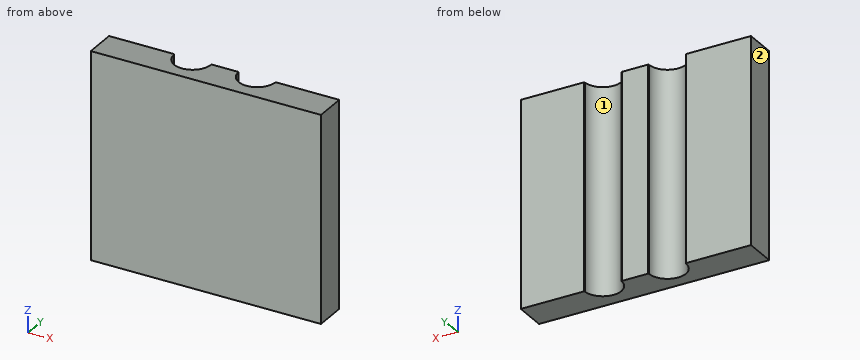
```python
from build123d import *

# Parameters (mm, degrees)
SKETCH1_W           = 38
SKETCH1_H           = 34
BOSS_EXTRUDE1_DEPTH = 2
BOSS_EXTRUDE2_DEPTH = 34
CHAMFER1_SIZE       = 0.1
CHAMFER1_SIZE_2     = 0.100939666
CHAMFER1_SIZE_3     = 0.096996068


with BuildPart() as part:
    # Sketch1 → Boss-Extrude1 (new body)
    with BuildSketch(Plane(origin=(0, 0, 0), x_dir=(1, 0, 0), z_dir=(0, 1, 0))):
        Rectangle(SKETCH1_W, SKETCH1_H)
    extrude(amount=BOSS_EXTRUDE1_DEPTH)

    # Sketch2 → Boss-Extrude2 (add, through all)
    with BuildSketch(Plane.XY.offset(17)):
        with BuildLine():
            Line((-2.101169585, 5.192456713), (2.394541693, 5.192456713))
            ThreePointArc((2.394541693, 5.192456713), (5.447861319, 2.177768465), (8.494206352, 5.199504374))
            Line((8.494206352, 5.199504374), (19, 5.199504374))
            Line((19, 5.199504374), (19, 1.662378765))
            Line((19, 1.662378765), (-19, 1.662378765))
            Line((-19, 1.662378765), (-19, 5.198537403))
            Line((-19, 5.198537403), (-8.197951747, 5.198537403))
            ThreePointArc((-8.197951747, 5.198537403), (-5.152701361, 2.046490686), (-2.101169585, 5.192456713))
        make_face()
    extrude(amount=-BOSS_EXTRUDE2_DEPTH)

    # Chamfer1
    # the kernel refuses this chamfer: 0.101178115, 0.100939666, 0.1, 0.096996068, 0.096814929 mm, written as the material it takes off along each edge
    with BuildSketch(Plane(origin=(2.394541693, 5.192456713, 17.264875528), x_dir=(0.028454787424249305, -0.9995950805564424, 0), z_dir=(0, 0, -1))) as chamfer1_piece_1:
        with BuildLine():
            Line((0.102971734, 0), (-CHAMFER1_SIZE * 0.0284547874242, CHAMFER1_SIZE * 0.999595080556))
            Line((-CHAMFER1_SIZE * 0.0284547874242, CHAMFER1_SIZE * 0.999595080556), (0, 0))
            ThreePointArc((0, 0), (0.052957758, 0.000434232), (0.102971734, 0))
        make_face()
    extrude(amount=34.529751055, mode=Mode.SUBTRACT)
    with BuildSketch(Plane(origin=(8.494206352, 5.199504374, 17.261624735), x_dir=(1, 0, 0), z_dir=(0, 0, -1))) as chamfer1_piece_2:
        with BuildLine():
            Line((CHAMFER1_SIZE_2 * 0.999999995384, 0), (-0.002638157, 0.10167581))
            ThreePointArc((-0.002638157, 0.10167581), (-0.000933226, 0.052300381), (0, 0))
            Line((0, 0), (CHAMFER1_SIZE_2 * 0.999999995384, 0))
        make_face()
    extrude(amount=34.52324947, mode=Mode.SUBTRACT)
    with BuildSketch(Plane(origin=(-8.197951747, 5.198537403, 17.257168299), x_dir=(-0.017346814306717553, -0.9998495326964995, 0), z_dir=(0, 0, -1))) as chamfer1_piece_3:
        with BuildLine():
            Line((0.098309437, 0), (CHAMFER1_SIZE * 0.0173468143067, CHAMFER1_SIZE * 0.999849532696))
            Line((CHAMFER1_SIZE * 0.0173468143067, CHAMFER1_SIZE * 0.999849532696), (0, 0))
            ThreePointArc((0, 0), (0.050545023, 0.000395805), (0.098309437, 0))
        make_face()
    extrude(amount=34.514336598, mode=Mode.SUBTRACT)
    with BuildSketch(Plane(origin=(-2.101169585, 5.192456713, 17.261555472), x_dir=(1, 0, 0), z_dir=(0, 0, -1))) as chamfer1_piece_4:
        with BuildLine():
            Line((CHAMFER1_SIZE_3 * 0.999999996404, 0), (0.001504787, 0.101698897))
            ThreePointArc((0.001504787, 0.101698897), (0.001197292, 0.052281476), (0, 0))
            Line((0, 0), (CHAMFER1_SIZE_3 * 0.999999996404, 0))
        make_face()
    extrude(amount=34.523110943, mode=Mode.SUBTRACT)


solid = part.part
```
The listing builds one solid part. Answer for the finished solid, in the listing's coordinates (mm). Face numbers are marked on the shaded views. Coordinates: 2 decimals unless noted, no trailing zeros. Write each loop counter-clockwise with the first axis right and the second up, starting at its lowest first coordinate (ties: lowest second). Pieces come first, ordered by that corner, then holes. Notation, with made-up numbers: (-14.5, -4) - (16.5, -4) arc R15 ccw to (16.5, 18) - close; hole circle Ø10 at (-20.5, 41.5). An arc over 180 degrees is marked (long way). Return JSON: item names as keys, results as strings. Group by question number.
Q1. The part is cut by section D-D on x = 3.5. Write down the section's boundary in (y, z).
Q2. Find the intervals of material crossed by line 1 along X through (y, z) = (4.85, 14.5); line 2 along X through (y, z) = (4.45, 3); line 3 along Y through (x, z) = (1, 7), in increasing order. Write a range as [from, to].
Q3. The part is cut by section B-B on z = 6.5. Write down the section's boundary in (x, y).
Q4. For a pull along X with two mould halves and no side action, classify the marked faces 1 and 2 as +X half, -X half, draft (parallel to the pull), parting line (faces both ways), or undercut.
Q5. The part is cut by section C-C on x = -6. Write down the section's boundary in (y, z), and give its area (3 significant figures).
Q6. The part is cut by section A-A on y = 3.65. Write down the section's boundary in (x, z).
Q7. Flat-ended cylindrical pins translate along their axes: pin 1 Ø4.5 at (x, z) = (-0.5, -3.5) entering from +Y; pin 2 Ø2 at (x, z) = (6, -12.5) entering from +Y. Find the tip coordinate at first contact, or state that the pin passes through.
Evaluation:
{
 "1": {"outline": "(0, -17) - (2.88, -17) - (2.88, 17) - (0, 17) - close"},
 "2": {"line 1": "x = [-19, -8.19], [-2.11, 2.42], [8.47, 19]", "line 2": "x = [-19, -8.13], [-2.17, 2.5], [8.39, 19]", "line 3": "y = [0, 5.19]"},
 "3": {"outline": "(-19, 0) - (19, 0) - (19, 5.2) - (8.6, 5.2) - (8.49, 5.1) arc R3.05 cw to (2.4, 5.09) - (2.29, 5.19) - (-2, 5.19) - (-2.1, 5.09) arc R3.05 cw to (-8.2, 5.1) - (-8.3, 5.2) - (-19, 5.2) - close"},
 "4": {"face 1": "undercut", "face 2": "-X half"},
 "5": {"outline": "(0, -17) - (2.17, -17) - (2.17, 17) - (0, 17) - close", "area": "73.7 mm2"},
 "6": {"outline": "(-19, -17) - (-7.83, -17) - (-7.83, 17) - (-19, 17) - close; (-2.46, -17) - (2.83, -17) - (2.83, 17) - (-2.46, 17) - close; (8.05, -17) - (19, -17) - (19, 17) - (8.05, 17) - close"},
 "7": {"pin 1": "stops at y = 5.19", "pin 2": "stops at y = 2.6"}
}
